Here's how the part is built. I have some questions about the finished solid (model axes, mm). A direction names the side the tool comes from. Round coordinates to 2 decimals unless told otherwise and drop trailing zeros. Write each loop counter-clockwise with the first axis right and the second up, starting at its lowest first coordinate (ties: lowest second). Pieces come first, ordered by that corner, then holes. Notation, with made-up numbers: (-36.75, 28.25) - (18.25, 28.25) arc R14 ccw to (18.25, 52.25) - close; hole circle Ø5 at (3.25, 44.25). An arc over 180 degrees is marked (long way). Write item = value, one per line. Start each with the question number.
Item 1: If we section it at A-A (y = 0): Please give me the cut outline in (x, z).
Item 2: For P1, Ø3, axis at x = 0, y = -16, coming from the +Z side; P2, Ø3, axis at x = 0.5, y = 9.5, coming from the -Z side; P3, Ø6, axis at x = -5.5, z = -7, coming from the +Y side, each with a flat end and sliding along its axis, tell me the tip position at first contact or that it passes through.
Item 3: If I drill on line 1 along X through (y, z) = (5.5, 19); line 2 along Z through (x, y) = (-6.5, -9); line 3 along Y through (x, z) = (-4.5, 2), over which ranges is the centre line in solid material (lowest first)? Write a range as [from, to].
Item 4: Which directions (+Z, -Z, +X, -X, +Y, -Y) give clear straight access to the entire face, cutting with the end or side of a thin tool? Please do faces 1 (the face through (0, -16, -20)), 2 (the face through (-7.01, 15.62, -3.47)), 3 (the face through (-6, 16.2, 1.5)).
Item 5: Thinking about a two-plate mould opening in Y: for faces 4 (the face through (-5.612, -6.637, 21.077)), 5 (the face through (2, -4, -24)), 6 (the face through (-2.465, -7.509, 23.846)), which applies, pulls with the +Y half, pulls with the -Y half, needs draft (parallel to the pull), parting line crosses it, or undercut?
Item 6: If we section it at C-C (x = -2): Please give me the cut outline in (y, z), and give its area (3 significant figures).
Item 7: If we section it at D-D (x = 1): Please give me the cut outline in (y, z).
```python
from build123d import *

# Parameters (mm, degrees)
SFAZOWANIE1_SIZE  = 3
SFAZOWANIE1_SIZE2 = 0.5


with BuildPart() as part:
    # Szkic1 → Obrót1 (revolve)
    with BuildSketch(Plane.XY, mode=Mode.PRIVATE) as obr_t1_sk:
        Polygon((0, 26.5), (2, 26.5), (2, 24), (-6, 22), (-6, 16), (-8, 16), (-8, 25), (0, 25), align=None)
    revolve(obr_t1_sk.sketch.rotate(Axis((-21.448486922, 0, 0), (1, 0, 0)), 90), axis=Axis((-21.448486922, 0, 0), (1, 0, 0)))

    # Sfazowanie1
    sfazowanie1_edges = [part.edges().sort_by_distance(p)[0] for p in [
        (-8, 0, -25),
    ]]
    sfazowanie1_side = [part.faces().sort_by_distance(p)[0] for p in [
        (-4, 0, -25),
    ]]
    chamfer(sfazowanie1_edges, length=SFAZOWANIE1_SIZE, length2=SFAZOWANIE1_SIZE2, reference=sfazowanie1_side[0])


solid = part.part
```
Reply:
q1.outline = (-8, -24.5) - (-5, -25) - (0, -25) - (0, -26.5) - (2, -26.5) - (2, -24) - (-6, -22) - (-6, -16) - (-8, -16) - close; (-8, 16) - (-6, 16) - (-6, 22) - (2, 24) - (2, 26.5) - (0, 26.5) - (0, 25) - (-5, 25) - (-8, 24.5) - close
q2.P1 = 22.18
q2.P2 = -25.26
q2.P3 = 24.67
q3.line_1 = [-8, -6]
q3.line_2 = [-23.06, -13.23], [13.23, 23.06]
q3.line_3 = [-24.92, -22.29], [22.29, 24.92]
q4.face_1 = -X
q4.face_2 = +X, -X
q4.face_3 = +X
q5.face_4 = undercut
q5.face_5 = needs draft
q5.face_6 = parting line crosses it
q6.outline = circle Ø50 at (0, 0); hole circle Ø46 at (0, 0)
q6.area = 302 mm2
q7.outline = circle Ø53 at (0, 0); hole circle Ø47.5 at (0, 0)
